Part model, mm, in its own coordinate system. Round coordinates to 2 decimals unless told otherwise and drop trailing zeros. Write each loop counter-clockwise with the first axis right and the second up, starting at its lowest first coordinate (ties: lowest second). Pieces come first, ordered by that corner, then holes. Notation, with made-up numbers: M 7,50 L 32,50 A17 cw 32,54 Z; hole C 49.25,15.5 d5. An arc over 180 degrees is marked long. Use a Markdown table: item, result. Add a question column.
1) Slice it at D-D on x = 8. Write the cut outline in (y, z).
2) Drop flat-ended pins along their axis: P1, Ø1.5, axis at y = -1, z = -36.5, coming from the +X side; P2, Ø1.5, axis at x = 8.5, y = 2.5, coming from the -Z side; P3, Ø1, axis at y = -1, z = -3, coming from the +X side; P4, Ø4, axis at x = 4.2, z = -80.75, coming from the +Y side. Give the stop position or say it passes through.
3) Slice it at B-B on z = -15.75. Write the cut outline in (x, y).
4) Slice it at A-A on x = 4.2. Write the cut outline in (y, z).
5) Wall check: probe 1 along Z at (x, y) = (4.2, 3); probe 2 along Z at (x, y) = (3.5, 2.5); probe 3 along Z at (x, y) = (3.75, -0.55). Give the ranges that are in metal, low to high.
6) Slice it at C-C on z = -62.5. Write the cut outline in (x, y).
```python
from build123d import *

# Parameters (mm, degrees)
EXTRUDE_1_DEPTH          = 96.5
CHAMFER_1_SIZE           = 1
CHAMFER_2_SIZE           = 1
CUT_EXTRUDE_1_DEPTH      = 97.93327602
CUT_EXTRUDE_1_DEPTH_BACK = 10
SKETCH_2_R               = 1.2
SKETCH_2_3_R             = 2.05
CUT_EXTRUDE_2_DEPTH      = 2
CHAMFER_3_SIZE           = 2
SKETCH_3_W               = 1.8
SKETCH_3_H               = 7.4
CUT_EXTRUDE_3_DEPTH      = 1.9
CHAMFER_4_SIZE           = 0.2
CHAMFER_5_SIZE           = 0.6
SKETCH_4_W               = 3.9
SKETCH_4_H               = 7.9
EXTRUDE_2_DEPTH          = 2
CHAMFER_6_SIZE           = 0.4
EXTRUDE_3_DEPTH          = 96.5


with BuildPart() as part:
    # 草图1 → 凸台-拉伸1 (new body)
    with BuildSketch(Plane.XY):
        Polygon((0, 0), (7, 0), (7, 4), (0, 4), (-1.8, 4), (-1.8, -1.9), (0, -1.9), align=None)
    extrude(amount=-EXTRUDE_1_DEPTH)

    # 倒角1
    chamfer_1_edges = [part.edges().sort_by_distance(p)[0] for p in [
        (7, 0, -48.25),
    ]]
    chamfer(chamfer_1_edges, length=CHAMFER_1_SIZE)

    # 倒角2
    chamfer_2_edges = [part.edges().sort_by_distance(p)[0] for p in [
        (7, 4, -48.25),
    ]]
    chamfer(chamfer_2_edges, length=CHAMFER_2_SIZE)

    # 草图2 → 切除-拉伸1 (cut, two sides: drawn at the far end of the back side and taken through both)
    with BuildSketch(Plane(origin=(0, 4, 0), x_dir=(1, 0, 0), z_dir=(0, 1, 0)).offset(-CUT_EXTRUDE_1_DEPTH_BACK)):
        with Locations(Location((4.2, 80.75, 0), (0, 0, 90))):
            Circle(SKETCH_2_R)
        with Locations(Location((4.2, 15.75, 0), (0, 0, 90))):
            Circle(SKETCH_2_R)
    extrude(amount=CUT_EXTRUDE_1_DEPTH + CUT_EXTRUDE_1_DEPTH_BACK, mode=Mode.SUBTRACT)

    # 草图2<3> → 切除-拉伸2 (cut)
    with BuildSketch(Plane(origin=(0, 4, 0), x_dir=(1, 0, 0), z_dir=(0, 1, 0))):
        with Locations(Location((4.2, 80.75, 0), (0, 0, 270))):
            Circle(SKETCH_2_3_R)
        with Locations(Location((4.2, 15.75, 0), (0, 0, 270))):
            Circle(SKETCH_2_3_R)
    extrude(amount=-CUT_EXTRUDE_2_DEPTH, mode=Mode.SUBTRACT)

    # 倒角3
    chamfer_3_edges = [part.edges().sort_by_distance(p)[0] for p in [
        (-1.8, 4, -48.25),
    ]]
    chamfer(chamfer_3_edges, length=CHAMFER_3_SIZE)

    # 草图3 → 切除-拉伸3 (cut)
    with BuildSketch(Plane.XZ.offset(1.9)):
        with Locations((-0.9, -92.8)):
            Rectangle(SKETCH_3_W, SKETCH_3_H)
        with Locations((-0.9, -3.7)):
            Rectangle(SKETCH_3_W, SKETCH_3_H)
    extrude(amount=-CUT_EXTRUDE_3_DEPTH, mode=Mode.SUBTRACT)

    # 倒角4
    chamfer_4_edges = [part.edges().sort_by_distance(p)[0] for p in [
        (-1.8, -1.9, -48.25),
        (0, -1.9, -48.25),
        (-1.8, -0.95, -89.1),
        (0, -0.95, -89.1),
        (-1.8, 0, -92.8),
        (-1.8, -0.95, -7.4),
        (0, -0.95, -7.4),
        (-1.8, 0, -3.7),
    ]]
    chamfer(chamfer_4_edges, length=CHAMFER_4_SIZE)

    # 倒角5
    # the kernel refuses this chamfer: 0.6 mm, written as the material it takes off along each edge
    with BuildSketch(Plane(origin=(1.343009793, -1.9, -89.1), x_dir=(0, 0.9996219169112965, -0.027495876610595982), z_dir=(-1, 0, 0))) as chamfer_5_piece_1:
        Polygon((CHAMFER_5_SIZE * 0.999621916911, -CHAMFER_5_SIZE * 0.0274958766106), (-CHAMFER_5_SIZE * 0.0274958766106, -CHAMFER_5_SIZE * 0.999621916911), (0, 0), align=None)
    extrude(amount=4.486019586, mode=Mode.SUBTRACT)
    with BuildSketch(Plane(origin=(1.343009793, -1.9, -7.4), x_dir=(0, 0.9996219169112968, 0.027495876610585925), z_dir=(-1, 0, 0))) as chamfer_5_piece_2:
        Polygon((CHAMFER_5_SIZE * 0.999621916911, CHAMFER_5_SIZE * 0.0274958766106), (-CHAMFER_5_SIZE * 0.0274958766106, CHAMFER_5_SIZE * 0.999621916911), (0, 0), align=None)
    extrude(amount=4.486019586, mode=Mode.SUBTRACT)

    # 草图4 → 凸台-拉伸2 (add)
    with BuildSketch(Plane.XZ):
        with Locations((4.05, -92.55)):
            Rectangle(SKETCH_4_W, SKETCH_4_H)
        with Locations((4.05, -3.95)):
            Rectangle(SKETCH_4_W, SKETCH_4_H)
    extrude(amount=EXTRUDE_2_DEPTH)

    # 倒角6
    chamfer_6_edges = [part.edges().sort_by_distance(p)[0] for p in [
        (6, -1, -88.6),
        (6, -1, -7.9),
    ]]
    chamfer(chamfer_6_edges, length=CHAMFER_6_SIZE)

    # 草图5 → 凸台-拉伸3 (add)
    with BuildSketch(Plane.XY):
        Polygon((7, 3), (9.4, 0.6), (9.4, 0), (7, 0), (6.5, 0.5), (7, 1), align=None)
    extrude(amount=-EXTRUDE_3_DEPTH)


solid = part.part
```
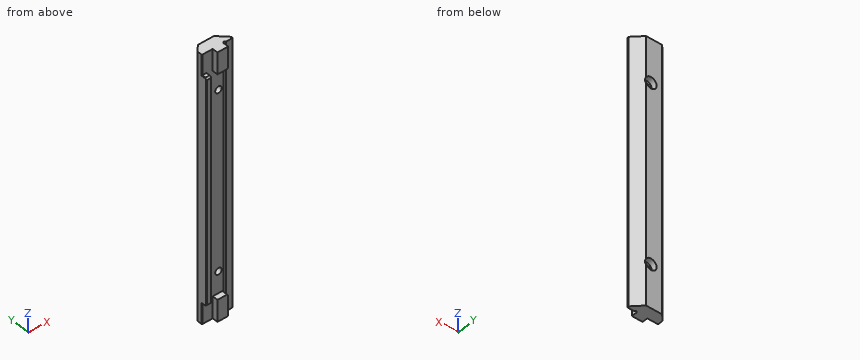
Entries:
| question | item | result |
|---|---|---|
| 1 | outline | M 0,-96.5 L 2,-96.5 L 2,0 L 0,0 Z |
| 2 | P1 | stops at x = 0 |
| 2 | P2 | stops at z = -96.5 |
| 2 | P3 | stops at x = 6 |
| 2 | P4 | stops at y = 2 |
| 3 | outline | M -1.8,-1.7 L -1.6,-1.9 L -0.2,-1.9 L 0,-1.7 L 0,0 L 3,0 L 3,2 L 2.15,2 L 2.15,4 L 0.2,4 L -1.8,2 Z; M 5.4,0 L 6,0 L 6.5,0.5 L 7,0 L 9.4,0 L 9.4,0.6 L 6.25,3.75 L 6.25,2 L 5.4,2 Z |
| 4 | outline | M -2,-96.5 L 4,-96.5 L 4,-82.8 L 2,-82.8 L 2,-81.95 L 0,-81.95 L 0,-88.6 L -2,-88.6 Z; M -2,-7.9 L 0,-7.9 L 0,-14.55 L 2,-14.55 L 2,-13.7 L 4,-13.7 L 4,0 L -2,0 Z; M 0,-79.55 L 2,-79.55 L 2,-78.7 L 4,-78.7 L 4,-17.8 L 2,-17.8 L 2,-16.95 L 0,-16.95 Z |
| 5 | probe 1 | z = -96.5 to -82.8, -78.7 to -17.8, -13.7 to 0 |
| 5 | probe 2 | z = -96.5 to -82.68, -78.82 to -17.68, -13.82 to 0 |
| 5 | probe 3 | z = -96.5 to -88.6, -7.9 to 0 |
| 6 | outline | M -1.8,-1.7 L -1.6,-1.9 L -0.2,-1.9 L 0,-1.7 L 0,0 L 6,0 L 6.5,0.5 L 7,0 L 9.4,0 L 9.4,0.6 L 6,4 L 0.2,4 L -1.8,2 Z |
